Read the model definition and answer for the solid it produces. Units are mm, in the model's axes. Coordinates: 2 decimals unless noted, no trailing zeros. Loops run counter-clockwise (first coordinate to the right, second up) from the corner with the lowest first, then second, coordinate; pieces in that order, holes last. Notation, with made-up numbers: M 80,10 L 134,10 A19 cw 134,34 Z; hole C 41.5,35.25 d6. An arc over 180 degrees is marked long. One line per item, written item: value. Start each with the question number.
1. Consider probe 1 along X at (y, z) = (1.5, -102); probe 2 along Y at (x, z) = (4, 627); probe 3 along Y at (x, z) = (45, 1071). Determine where each line is inside the solid, lowest interval first.
2. The part is cut by section B-B (y = 3). Write down the section's boundary in (x, z), then the cut area to 3 significant figures.
3. A flat-ended cylindrical pin translates along its axis: pin 1 (10 mm diameter, centred on x = 28, y = 19.5, fed in from +Z). Find the tip coordinate at first contact, or state that the pin passes through.
4. The part is cut by section C-C (x = -3.5). Write down the section's boundary in (y, z), then the cut area to 3 significant figures.
5. The part is cut by section A-A (z = 25.5). Write down the section's boundary in (x, y), then the cut area to 3 significant figures.
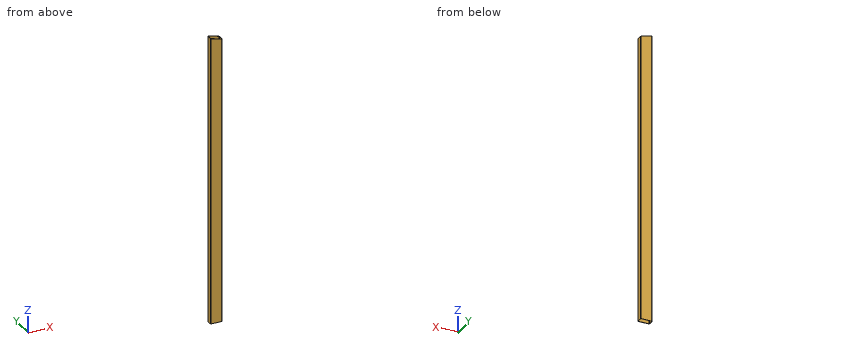
```python
from build123d import *

# Parameters (mm, degrees)
F1_DEPTH = 1250
F3_DEPTH = 50.001


with BuildPart() as f1:
    # F0 (on Top) → F1 (new body, symmetric)
    with BuildSketch(Plane.XY):
        with BuildLine():
            Line((44, 25), (-44, 25))
            ThreePointArc((-44, 25), (-48.2426406871, 23.2426406871), (-50, 19))
            Line((-50, 19), (-50, -19))
            ThreePointArc((-50, -19), (-48.2426406871, -23.2426406871), (-44, -25))
            Line((-44, -25), (44, -25))
            ThreePointArc((44, -25), (48.2426406871, -23.2426406871), (50, -19))
            Line((50, -19), (50, 19))
            ThreePointArc((50, 19), (48.2426406871, 23.2426406871), (44, 25))
        make_face()
        with BuildLine():
            ThreePointArc((-48, 19), (-46.8284271247, 21.8284271247), (-44, 23))
            Line((-44, 23), (44, 23))
            ThreePointArc((44, 23), (46.8284271247, 21.8284271247), (48, 19))
            Line((48, 19), (48, -19))
            ThreePointArc((48, -19), (46.8284271247, -21.8284271247), (44, -23))
            Line((44, -23), (-44, -23))
            ThreePointArc((-44, -23), (-46.8284271247, -21.8284271247), (-48, -19))
            Line((-48, -19), (-48, 19))
        make_face(mode=Mode.SUBTRACT)
    extrude(amount=F1_DEPTH, both=True)

    # F2 (on face) → F3 (cut, through all)
    with BuildSketch(Plane.XZ.offset(25)):
        Polygon((50, 1223.2050807569), (50, 1250), (44, 1250), (44, 1224.8127759115), align=None)
        Polygon((44, 1224.8127759115), (44, 1250), (-44, 1250), (-44, 1248.3923048454), align=None)
        Polygon((-44, 1248.3923048454), (-44, 1250), (-50, 1250), align=None)
    extrude(amount=-F3_DEPTH, mode=Mode.SUBTRACT)


solid = f1.part
```
Answer block:
1. probe 1: x = -50 to -48, 48 to 50
1. probe 2: y = -25 to -23, 23 to 25
1. probe 3: y = -24.92 to -22.87, 22.87 to 24.92
2. outline: M -50,-1250 L -48,-1250 L -48,1249.46 L -50,1250 Z; M 48,-1250 L 50,-1250 L 50,1223.21 L 48,1223.74 Z
2. area: 9,950 mm2
3. pin 1: stops at z = 1230.06
4. outline: M -25,-1250 L -23,-1250 L -23,1237.54 L -25,1237.54 Z; M 23,-1250 L 25,-1250 L 25,1237.54 L 23,1237.54 Z
4. area: 9,950 mm2
5. outline: M -50,-19 A6 ccw -44,-25 L 44,-25 A6 ccw 50,-19 L 50,19 A6 ccw 44,25 L -44,25 A6 ccw -50,19 Z; hole M -48,-19 A4 ccw -44,-23 L 44,-23 A4 ccw 48,-19 L 48,19 A4 ccw 44,23 L -44,23 A4 ccw -48,19 Z
5. area: 567 mm2
